Study the drawing (mm; zero at the part's minimum x, y, z) and answer. Give positions to 0.01 mm unless a question says otherwise; leave off trailing zeros. Write each loop counter-clockwise with the first axis right and the second up, starting at its lowest first coordinate (ties: lowest second). Pieces come first, ordered by that corner, then holes.
1) Straight lines are drawn through the part: probe 1 along X at (y, z) = (24.5, 36) (1 decimal); probe 2 along Y at (x, z) = (40, 24); probe 3 along Z at (x, y) = (90, 18.5). For each, find the intervals that lie inside material, in ascending order.
2) Find section D-D (y = 20). Count the separate pieces of the cut face and the enclosed holes in it, plus the area to 3 significant figures.
3) Given pin 1 Ø5 at (x, z) = (133, 65) entering from +Y; pin 2 Ø8 at (x, z) = (109, 81) entering from -Y; pin 3 Ø1.5 at (x, y) = (77.5, 24) entering from +Z (1 decimal), each flat-ended and moving along its own axis, determine where each tip first touches the part or whether it passes through.
4) Find section A-A (x = 11.5). Determine the outline of the cut face in (y, z) (1 decimal).
5) Determine the mould class of the marked faces 1, 2, 3 and 4 for opening direction X: pulls with the +X half, pulls with the -X half, needs draft (parallel to the pull), parting line crosses it, or undercut.
6) Find section C-C (x = 133.5). Determine the outline of the cut face in (y, z), plus the area to 3 significant figures.
7) Find section B-B (z = 12.5). Determine the outline of the cut face in (x, y) (1 decimal).
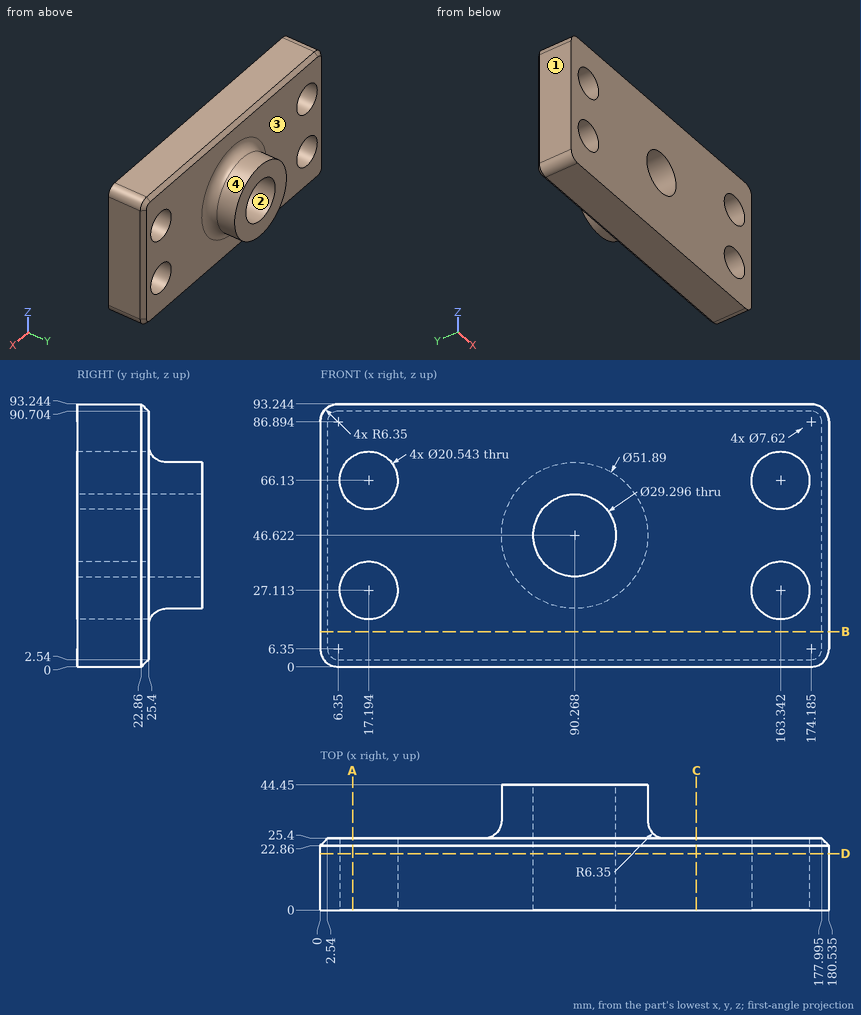
Results:
1. probe 1: x = 1.6 to 12, 22.3 to 80.2, 100.4 to 158.2, 168.5 to 178.9
1. probe 2: y = 0 to 25.4
1. probe 3: z = 0 to 31.98, 61.27 to 93.24
2. separate pieces: 1
2. enclosed holes: 5
2. area: 14,800 mm2
3. pin 1: stops at y = 25.4
3. pin 2: stops at y = 0
3. pin 3: stops at z = 92.9
4. outline: (0, 0) - (22.9, 0) - (25.4, 2.5) - (25.4, 18.6) - (0, 18.6) - close; (0, 35.7) - (25.4, 35.7) - (25.4, 57.6) - (0, 57.6) - close; (0, 74.7) - (25.4, 74.7) - (25.4, 90.7) - (22.9, 93.2) - (0, 93.2) - close
5. face 1: pulls with the -X half
5. face 2: undercut
5. face 3: needs draft
5. face 4: parting line crosses it
6. outline: (0, 0) - (22.86, 0) - (25.4, 2.54) - (25.4, 90.7) - (22.86, 93.24) - (0, 93.24) - close
6. area: 2,360 mm2
7. outline: (0, 0) - (180.5, 0) - (180.5, 22.9) - (178, 25.4) - (2.5, 25.4) - (0, 22.9) - close
